Verification items for the finished model (mm, model axes). A direction names the side the tool comes from. Coordinates: 2 decimals unless noted, no trailing zeros. Loops run counter-clockwise (first coordinate to the right, second up) from the corner with the lowest first, then second, coordinate; pieces in that order, holes last. Notation, with made-up numbers: (-13, 37.5) -> (11, 37.5) arc R17 ccw to (11, 45.5) -> close; hole circle Ø10 at (18, 30). An arc over 180 degrees is marked (long way). Write item = value, one per line.
```python
from build123d import *

# Parameters (mm, degrees)
F1_DEPTH = 50
F2_R     = 4
F3_DEPTH = 15


with BuildPart() as f1:
    # F0 (on Right) → F1 (new body)
    with BuildSketch(Plane.YZ):
        with BuildLine():
            Line((-7.864183, 0), (-4.410664, -19.585883))
            ThreePointArc((-4.410664, -19.585883), (0, -70), (4.410664, -19.585883))
            Line((4.410664, -19.585883), (7.864183, 0))
            Line((7.864183, 0), (-7.864183, 0))
        make_face()
    extrude(amount=F1_DEPTH)

    # F2 (on face) → F3 (join)
    with BuildSketch(Plane.XY):
        with Locations((25, 0)):
            Circle(F2_R)
    extrude(amount=F3_DEPTH)


solid = f1.part
```
1) Material ranges on line 1 (Z direction, x = 14, y = 10.5); line 2 (Z direction, x = 37, y = -17); line 3 (Y direction, x = 44, z = -13), recorded low to high.
Ans:
line_1 = -67.73 to -21.47
line_2 = -63.47 to -25.73
line_3 = -5.57 to 5.57
2) Tool access check on faces 4 (the face through (24.65, 6.113, -9.93)), 5 (the face through (24.65, -1.05, -69.98)). Record the directions out of +Z, -Z, +X, -X, +Y, -Y that give a thin tool (end or side, any length) a straight path to the whole face; none if there is none.
Ans:
face_4 = +X, -X, +Y
face_5 = +X, -X
3) Sectioned sample at B-B, the plane y = 0. Record the cut outline in (x, z), plus the area to 3 significant figures.
Ans:
outline = (0, -70) -> (50, -70) -> (50, 0) -> (29, 0) -> (29, 15) -> (21, 15) -> (21, 0) -> (0, 0) -> close
area = 3,620 mm2
4) Sectioned sample at D-D, the plane z = -51. Record the cut outline in (x, y), plus the area to 3 significant figures.
Ans:
outline = (0, -24.58) -> (50, -24.58) -> (50, 24.58) -> (0, 24.58) -> close
area = 2,460 mm2
5) Sectioned sample at C-C, the plane x = 40. Record the cut outline in (y, z), plus the area to 3 significant figures.
Ans:
outline = (-7.86, 0) -> (-4.41, -19.59) arc R25.4 ccw (long way) to (4.41, -19.59) -> (7.86, 0) -> close
area = 2,260 mm2
6) Depth check by flat-ended pin: pin 1 Ø1.5 at (x, z) = (35, -26) entering from -Y; pin 2 Ø4 at (x, z) = (14.5, -37) entering from +Y (3 decimals); pin 3 Ø10 at (x, z) = (35.5, -52.5) entering from +Y; pin 4 Ø8 at (y, z) = (-14.5, -16) entering from +X (3 decimals). Enter the tip coordinate at first touch or a pass-through.
Ans:
pin_1 = -18.07
pin_2 = 24.775
pin_3 = 25.23
pin_4 = through
7) Sectioned sample at A-A, the plane x = 25. Record the cut outline in (y, z).
Ans:
outline = (-7.86, 0) -> (-4.41, -19.59) arc R25.4 ccw (long way) to (4.41, -19.59) -> (7.86, 0) -> (4, 0) -> (4, 15) -> (-4, 15) -> (-4, 0) -> close
8) Release check for a two-part mould opening along Z. For faces 1 (the face through (25, 0, 15)), 2 (the face through (24.65, -6.16, -9.66)), 3 (the face through (21.8, -2.4, 7.4)) record: pulls with the +Z half, pulls with the -Z half, needs draft (parallel to the pull), parting line crosses it, or undercut.
Ans:
face_1 = pulls with the +Z half
face_2 = undercut
face_3 = needs draft
